from build123d import *

# Parameters (mm, degrees)
F0_R     = 37.5
F1_DEPTH = 3
F2_R     = 32.5
F2_R_2   = 31
F3_DEPTH = 25
F4_W     = 20
F4_H     = 33
F5_DEPTH = 25
F6_W     = 8.066451
F6_H     = 38.420005
F7_DEPTH = 25


with BuildPart() as f1:
    # F0 (on Top) → F1 (new body)
    with BuildSketch(Plane.XY):
        Circle(F0_R)
    extrude(amount=F1_DEPTH)

    # F2 (on face) → F3 (join)
    with BuildSketch(Plane(origin=(0, 0, 0), x_dir=(1, 0, 0), z_dir=(0, 0, -1))):
        Circle(F2_R)
        Circle(F2_R_2, mode=Mode.SUBTRACT)
    extrude(amount=F3_DEPTH)

    # F4 (on face) → F5 (cut)
    with BuildSketch(Plane.XY.offset(3)):
        Rectangle(F4_W, F4_H)
    extrude(amount=-F5_DEPTH, mode=Mode.SUBTRACT)

    # F6 (on face) → F7 (cut)
    with BuildSketch(Plane(origin=(0, 0, 0), x_dir=(1, 0, 0), z_dir=(0, 0, -1))):
        with Locations((36.533226, 0.501715)):
            Rectangle(F6_W, F6_H)
    extrude(amount=-F7_DEPTH, mode=Mode.SUBTRACT)


solid = f1.part
Verification items for the finished model (mm, model axes). A direction names the side the tool comes from. Round coordinates to 2 decimals unless told otherwise and drop trailing zeros. Loops run counter-clockwise (first coordinate to the right, second up) from the corner with the lowest first, then second, coordinate; pieces in that order, holes last. Notation, with made-up numbers: (18.25, 80.5) - (28.25, 80.5) arc R23 cw to (28.25, 111.5) - close; hole circle Ø8 at (83, 84.5). An arc over 180 degrees is marked (long way). Use a Markdown table: item, result. Add a question column.
1. Access from +Z, -Z, +X, -X, +Y, -Y to the whole of each face (thin tool, end or side, straight path). Record for faces 1 (the face through (-10, 0, 2)), 2 (the face through (29, 12, -25)), 3 (the face through (-4.036, -30.736, -12.325)).
2. Section check C-C, the plane z = -17. Record the boundary of the cut face in (x, y), plus the area to 3 significant figures.
3. Section check D-D, the plane x = -25.5. Record the boundary of the cut face in (y, z).
4. Thickness scan on probe 1 along Y at (x, z) = (0, -19.5); probe 2 along Z at (x, y) = (-7.5, -30). Record the ranges inside material, lowest first. Write a range as [from, to].
5. Gauge pin test, flat ends, axial feed: pin 1 (10 mm diameter, centred on y = 10.5, z = -7, fed in from -X); pin 2 (1.5 mm diameter, centred on x = 2.5, z = 2, fed in from +Y); pin 3 (3 mm diameter, centred on y = 8.5, z = -18, fed in from -X). Record the tip position at first contact, or that the pin passes through.
6. Release check for a two-part mould opening along X. For faces 4 (the face through (-37.475, 1.375, 1.479)), 5 (the face through (-31, -11, 0)), 6 (the face through (10, 0, 2)), 7 (the face through (32.5, 0, 1)) record: released by +X, released by -X, zero draft, split by the parting line, or undercut.
7. Section check A-A, the plane x = 0. Record the boundary of the cut face in (y, z).
8. Section check B-B, the plane y = -13.5. Record the boundary of the cut face in (x, z).
Checks:
| question | item | result |
|---|---|---|
| 1 | face 1 | +Z, -Z |
| 1 | face 2 | -Z, +X, -X, +Y, -Y |
| 1 | face 3 | -Z |
| 2 | outline | circle Ø65 at (0, 0); hole circle Ø62 at (0, 0) |
| 2 | area | 299 mm^2 |
| 3 | outline | (-27.5, 0) - (-20.15, 0) - (-20.15, -25) - (-17.63, -25) - (-17.63, 0) - (17.63, 0) - (17.63, -25) - (20.15, -25) - (20.15, 0) - (27.5, 0) - (27.5, 3) - (-27.5, 3) - close |
| 4 | probe 1 | y = [-32.5, -31], [31, 32.5] |
| 4 | probe 2 | z = [0, 3] |
| 5 | pin 1 | stops at x = -32.03 |
| 5 | pin 2 | stops at y = 37.46 |
| 5 | pin 3 | stops at x = -31.74 |
| 6 | face 4 | split by the parting line |
| 6 | face 5 | zero draft |
| 6 | face 6 | undercut |
| 6 | face 7 | released by +X |
| 7 | outline | (-37.5, 0) - (-32.5, 0) - (-32.5, -25) - (-31, -25) - (-31, 0) - (-16.5, 0) - (-16.5, 3) - (-37.5, 3) - close; (16.5, 0) - (31, 0) - (31, -25) - (32.5, -25) - (32.5, 0) - (37.5, 0) - (37.5, 3) - (16.5, 3) - close |
| 8 | outline | (-34.99, 0) - (-29.56, 0) - (-29.56, -25) - (-27.91, -25) - (-27.91, 0) - (-10, 0) - (-10, 3) - (-34.99, 3) - close; (10, 0) - (27.91, 0) - (27.91, -25) - (29.56, -25) - (29.56, 0) - (32.5, 0) - (32.5, 3) - (10, 3) - close |
